Design review of the part built by this model. Coordinates are the model's own, in mm. Face numbers are marked on the shaded views. A direction names the side the tool comes from. Coordinates: 2 decimals unless noted, no trailing zeros. Loops run counter-clockwise (first coordinate to the right, second up) from the corner with the lowest first, then second, coordinate; pieces in that order, holes last. Notation, with made-up numbers: (15, -14) -> (58, -14) arc R31 cw to (58, 11) -> close; hole circle Ø7 at (-10, -16). An arc over 180 degrees is marked (long way). Answer in a Markdown table with one row per item.
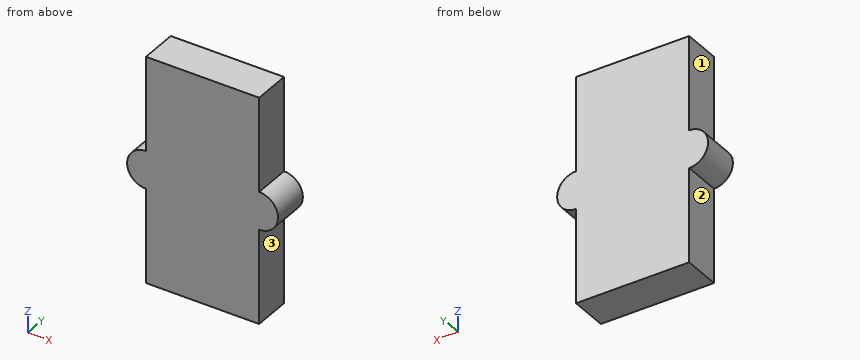
```python
from build123d import *

# Parameters (mm, degrees)
F1_DEPTH = 25.4


with BuildPart() as f1:
    # F0 (on Front) → F1 (new body)
    with BuildSketch(Plane.XZ):
        with BuildLine():
            Line((-38.1, -76.2), (38.1, -76.2))
            Line((38.1, -76.2), (38.1, -12.7))
            ThreePointArc((38.1, -12.7), (25.4, 0), (38.1, 12.7))
            Line((38.1, 12.7), (38.1, 76.2))
            Line((38.1, 76.2), (-38.1, 76.2))
            Line((-38.1, 76.2), (-38.1, 12.7))
            ThreePointArc((-38.1, 12.7), (-29.1197438789, 8.9802561211), (-25.4, 0))
            ThreePointArc((-25.4, 0), (-29.1197438789, -8.9802561211), (-38.1, -12.7))
            Line((-38.1, -12.7), (-38.1, -76.2))
        make_face()
        with BuildLine():
            ThreePointArc((38.1, 12.7), (25.4, 0), (38.1, -12.7))
            Line((38.1, -12.7), (38.1, 12.7))
        make_face()
        with BuildLine():
            Line((38.1, 12.7), (38.1, -12.7))
            ThreePointArc((38.1, -12.7), (47.0802561211, -8.9802561211), (50.8, 0))
            ThreePointArc((50.8, 0), (47.0802561211, 8.9802561211), (38.1, 12.7))
        make_face()
        with BuildLine():
            ThreePointArc((-38.1, 12.7), (-50.8, 0), (-38.1, -12.7))
            Line((-38.1, -12.7), (-38.1, 12.7))
        make_face()
        with BuildLine():
            Line((-38.1, 12.7), (-38.1, -12.7))
            ThreePointArc((-38.1, -12.7), (-29.1197438789, -8.9802561211), (-25.4, 0))
            ThreePointArc((-25.4, 0), (-29.1197438789, 8.9802561211), (-38.1, 12.7))
        make_face()
    extrude(amount=F1_DEPTH)


solid = f1.part
```
(1) Take a section at C-C on x = 44. Give the boundary of the cut face in (y, z), and give its area (3 significant figures).
Evaluation:
| item | result |
|---|---|
| outline | (-25.4, -11.25) -> (0, -11.25) -> (0, 11.25) -> (-25.4, 11.25) -> close |
| area | 571 mm² |
(2) Take a section at B-B on z = -26. Give the boundary of the cut face in (x, y).
Evaluation:
| item | result |
|---|---|
| outline | (-38.1, -25.4) -> (38.1, -25.4) -> (38.1, 0) -> (-38.1, 0) -> close |
(3) For pin 1 (1 mm diameter, centred on y = -12, z = 57, fed in from +X); pin 2 (8 mm diameter, centred on y = -16.5, z = 27.5, fed in from -X); pin 3 (1 mm diameter, centred on y = -20, z = -11, fed in from -X), all flat-tipped, find the tip position at first contact; note any pin that passes through.
Evaluation:
| item | result |
|---|---|
| pin 1 | stops at x = 38.1 |
| pin 2 | stops at x = -38.1 |
| pin 3 | stops at x = -45.24 |
(4) Take a section at A-A on y = -4.5. Give the boundary of the cut face in (x, z), and give its area (3 significant figures).
Evaluation:
| item | result |
|---|---|
| outline | (-38.1, -76.2) -> (38.1, -76.2) -> (38.1, -12.7) arc R12.7 ccw to (38.1, 12.7) -> (38.1, 76.2) -> (-38.1, 76.2) -> (-38.1, 12.7) arc R12.7 ccw to (-38.1, -12.7) -> close |
| area | 12,100 mm² |
(5) To check wall thickness, follow probe 1 along X at (y, z) = (-19, 42); probe 2 along X at (y, z) = (-4, -8). State the ranges of each line that lie inside material, in increasing order.
Evaluation:
| item | result |
|---|---|
| probe 1 | x = -38.1 to 38.1 |
| probe 2 | x = -47.96 to 47.96 |
(6) Tool access review of the marked faces 1, 2 and 3: name each direction out of +Z, -Z, +X, -X, +Y, -Y from which nothing blocks a thin tool from reaching the whole face with its end or side.
Evaluation:
| item | result |
|---|---|
| face 1 | +Z, -X, +Y, -Y |
| face 2 | -Z, -X, +Y, -Y |
| face 3 | -Z, +X, +Y, -Y |
